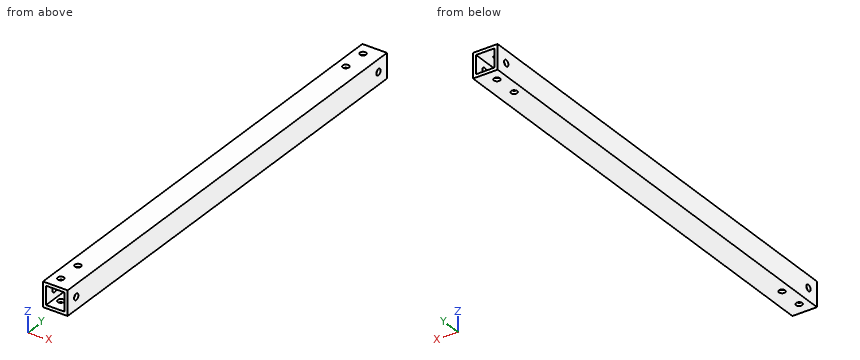
Autodesk Inventor part; units mm, degrees
ref_plane "YZ Plane" through (0, 0, 0) normal (1, 0, 0) x (0, 1, 0)
ref_plane "XZ Plane" through (0, 0, 0) normal (0, 1, 0) x (-1, 0, 0)
ref_plane "XY Plane" through (0, 0, 0) normal (0, 0, 1) x (1, 0, 0)
sketch "Sketch1" plane through (0, 0, 0) normal (0, 1, 0) x (-1, 0, 0)
  line L0 (0, 0) -> (25.4, 0)
  line L1 (25.4, 0) -> (25.4, 25.4)
  line L2 (25.4, 25.4) -> (0, 25.4)
  line L3 (0, 25.4) -> (0, 0)
  line L4 (22.225, 22.225) -> (22.225, 3.175)
  line L5 (22.225, 3.175) -> (3.175, 3.175)
  line L6 (3.175, 3.175) -> (3.175, 22.225)
  line L7 (3.175, 22.225) -> (22.225, 22.225)
  dimension "d0" = 25.4
  dimension "d1" = 25.4
  dimension "d2" = 3.175
extrude "Extrusion1" add sketch "Sketch1" along normal blind 472.9226
sketch "Sketch2" plane through (-25.4, 0, 0) normal (-1, 0, 0) x (0, 0, 1)
  circle A0 centre (12.7, 12.7) radius 3.175
  circle A1 centre (12.7, 460.2226) radius 3.175
  line L0 (22.225, 472.9226) -> (3.175, 472.9226)
  line L1 (25.4, 0) -> (25.4, 472.9226)
  line L2 (25.4, 0) -> (25.4, 472.9226)
  line L3 (0, 0) -> (25.4, 0)
  dimension "d5" = 6.35
  dimension "d6" = 6.35
  dimension "d7" = 12.7
  dimension "d8" = 12.7
  dimension "d9" = 12.7
  dimension "d10" = 12.7
extrude "Extrusion2" cut sketch "Sketch2" against normal blind 25.4
sketch "Sketch3" plane through (-25.4, 0, 25.4) normal (0, 0, 1) x (1, 0, 0)
  circle A0 centre (9.525, 460.2226) radius 3.175
  circle A1 centre (9.525, 434.8226) radius 3.175
  line L0 (0, 472.9226) -> (25.4, 472.9226)
  line L1 (0, 0) -> (0, 472.9226)
  circle A2 centre (9.525, 12.7) radius 3.175
  circle A3 centre (9.525, 38.1) radius 3.175
  line L2 (0, 0) -> (25.4, 0)
  dimension "d13" = 12.7
  dimension "d14" = 9.525
  dimension "d15" = 9.525
  dimension "d16" = 6.35
  dimension "d17" = 38.1
  dimension "d18" = 6.35
  dimension "d19" = 6.35
  dimension "d20" = 9.525
  dimension "d21" = 9.525
  dimension "d22" = 38.1
  dimension "d23" = 12.7
extrude "Extrusion3" cut sketch "Sketch3" against normal blind 25.4
properties part number "15102898-16-P-0206" material "Aluminum 6061"
Design review of the part built by this model. Coordinates are the model's own, in mm. Coordinates: 2 decimals unless noted, no trailing zeros. Order: outer loops, then holes, each group sorted by start corner. A loop starts at its lowest first (then second) coordinate and runs counter-clockwise, first axis right, second up.
1) Take a section at A-A, the plane x = -8. Give the boundary of the cut face in (y, z) (3 decimals), and give its area (3 significant figures).
2) Wall thickness on line 1 along X through (y, z) = (372, 4.25) (3 decimals); line 2 along Z through (x, y) = (-6, 401) (3 decimals); line 3 along Y through (x, z) = (-14.25, 2.5): over which ranges is each line inside the solid? List them lowest first.
3) Clearance check with a flat-ended pin moving along its axis: pin 1 (5 mm diameter, centred on x = -15.875, y = 38.1, fed in from -Z). State where the tip first meets the part, or that it passes through.
Returned:
1. outline: (0, 0) - (472.923, 0) - (472.923, 3.175) - (0, 3.175) - close; (0, 22.225) - (472.923, 22.225) - (472.923, 25.4) - (0, 25.4) - close
1. area: 3,000 mm2
2. line 1: x = -25.4 to -22.225, -3.175 to 0
2. line 2: z = 0 to 3.175, 22.225 to 25.4
2. line 3: y = 0 to 9.97, 15.43 to 35.37, 40.83 to 432.09, 437.55 to 457.49, 462.95 to 472.92
3. pin 1: passes through
